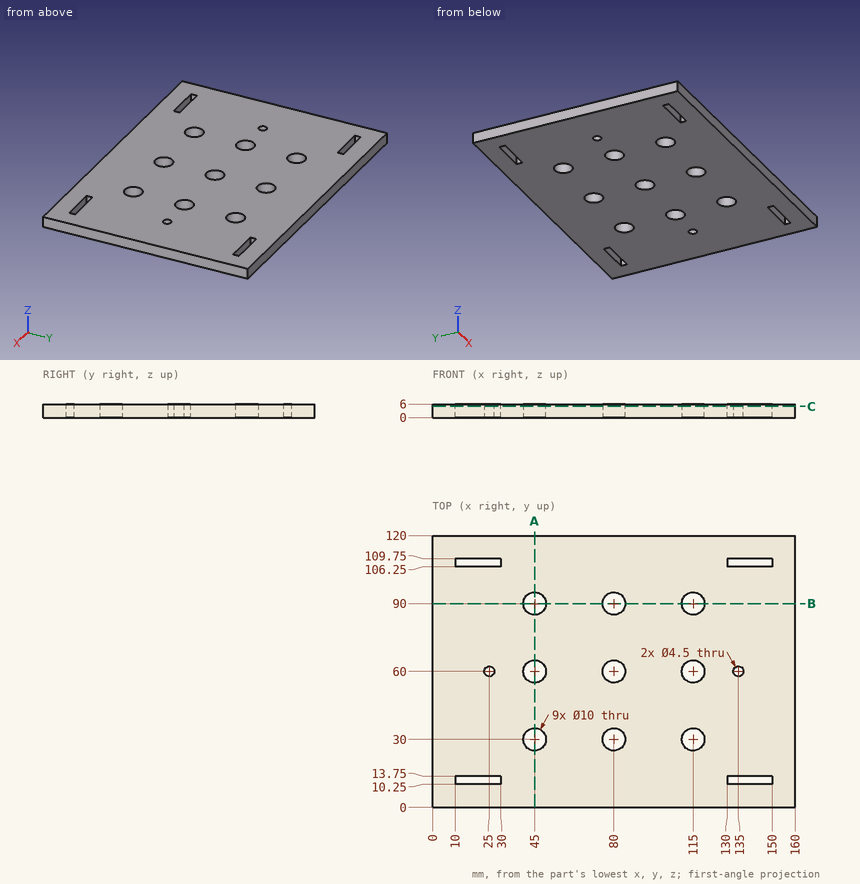
The figure shows three views and two pictorial views of one solid part (mm, origin at its lowest corner). Answer the questions. Coordinates: 2 decimals unless noted, no trailing zeros. Loops run counter-clockwise (first coordinate to the right, second up) from the corner with the lowest first, then second, coordinate; pieces in that order, holes last. Notation, with made-up numbers: (33.5, 33.25) -> (59.5, 33.25) arc R25 cw to (59.5, 47.25) -> close; hole circle Ø5 at (50, 55). An arc over 180 degrees is marked (long way). Write item = value, one per line. Start each with the question number.
1) Straight lines are drawn through the part: line 1 (X direction, y = 109, z = 1.1); line 2 (Y direction, x = 135, z = 3.2); line 3 (Y direction, x = 115, z = 3.75). For each, find the intervals that lie inside material, in ascending order. Write a range as from..to.
2) A cutting plane is placed at C-C (z = 4.95). Count the separate pieces of the cut face and the enclosed holes in it, then the cut area to 3 significant figures.
3) A cutting plane is placed at B-B (y = 90). Give the vertices of the cut face in (x, z), then the cut area to 3 significant figures.
4) A cutting plane is placed at A-A (x = 45). Give the vertices of the cut face in (y, z), then the cut area to 3 significant figures.
Responses:
q1.line_1 = 0..10, 30..130, 150..160
q1.line_2 = 0..10.25, 13.75..57.75, 62.25..106.25, 109.75..120
q1.line_3 = 0..25, 35..55, 65..85, 95..120
q2.separate_pieces = 1
q2.enclosed_holes = 15
q2.area = 18,200 mm²
q3.outline = (0, 0) -> (40, 0) -> (40, 6) -> (0, 6) -> close; (50, 0) -> (75, 0) -> (75, 6) -> (50, 6) -> close; (85, 0) -> (110, 0) -> (110, 6) -> (85, 6) -> close; (120, 0) -> (160, 0) -> (160, 6) -> (120, 6) -> close
q3.area = 780 mm²
q4.outline = (0, 0) -> (25, 0) -> (25, 6) -> (0, 6) -> close; (35, 0) -> (55, 0) -> (55, 6) -> (35, 6) -> close; (65, 0) -> (85, 0) -> (85, 6) -> (65, 6) -> close; (95, 0) -> (120, 0) -> (120, 6) -> (95, 6) -> close
q4.area = 540 mm²
